from build123d import *

# Parameters (mm, degrees)
CROQUIS2_R              = 1.5
CROQUIS2_R_2            = 1
CROQUIS2_W              = 3
CROQUIS2_H              = 2
SALIENTE_EXTRUIR1_DEPTH = 1


with BuildPart() as part:
    # Croquis2 → Saliente-Extruir1 (new body)
    with BuildSketch(Plane(origin=(0, 0, 0), x_dir=(1, 0, 0), z_dir=(0, 1, 0))):
        Polygon((38, 17), (-3, 17), (-3, 11), (3, 11), (3, 3), (-3, 3), (-3, -3), (15, -3), (15, -6), (20, -6), (20, -3), (38, -3), (38, 3), (32, 3), (32, 11), (38, 11), align=None)
        with Locations(Location((0, 14, 0), (0, 0, 270))):
            Circle(CROQUIS2_R, mode=Mode.SUBTRACT)
        with Locations(Location((0, 0, 0), (0, 0, 270))):
            Circle(CROQUIS2_R, mode=Mode.SUBTRACT)
        with Locations(Location((35, 0, 0), (0, 0, 270))):
            Circle(CROQUIS2_R, mode=Mode.SUBTRACT)
        with Locations(Location((35, 14, 0), (0, 0, 270))):
            Circle(CROQUIS2_R, mode=Mode.SUBTRACT)
        with Locations(Location((17.5, 7, 0), (0, 0, 270))):
            Circle(CROQUIS2_R_2, mode=Mode.SUBTRACT)
        with Locations((17.5, -4)):
            Rectangle(CROQUIS2_W, CROQUIS2_H, mode=Mode.SUBTRACT)
    extrude(amount=SALIENTE_EXTRUIR1_DEPTH)


solid = part.part
Read the model definition and answer for the solid it produces. Units are mm, in the model's axes. A direction names the side the tool comes from. Round coordinates to 2 decimals unless told otherwise and drop trailing zeros. Write each loop counter-clockwise with the first axis right and the second up, starting at its lowest first coordinate (ties: lowest second). Pieces come first, ordered by that corner, then holes. Notation, with made-up numbers: (35.5, 85.25) - (77.5, 85.25) arc R23 cw to (77.5, 94.25) - close; hole circle Ø11 at (87, -12). An arc over 180 degrees is marked (long way). One line per question, with ' | ' between items. Start each with the question number.
1. Each of these flat-tipped pins is pushed along its axis until it touches: pin 1 (1.8 mm diameter, centred on x = 17.5, z = -7, fed in from -Y); pin 2 (0.5 mm diameter, centred on y = 0.5, z = 4, fed in from +X); pin 3 (0.5 mm diameter, centred on x = 0, y = 0.5, fed in from +Z). Where does it stop, or does it pass through?
2. Section C-C (z = 0) is taken. Determine the outline of the cut face in (x, y).
3. Find the intervals of material crossed by probe 1 along X at (y, z) = (0.85, 0); probe 2 along X at (y, z) = (0.75, -7); probe 3 along Z at (x, y) = (1, 0.5), in increasing order. Write a range as [from, to].
4. Section A-A (x = 0) is taken. Determine the outline of the cut face in (y, z).
5. Section B-B (y = 0.2) is taken. Determine the outline of the cut face in (x, z), and give its area (3 significant figures).
6. For faces 1 (the face through (20, 0.5, 4.5)), 2 (the face through (0, 0.5, -11)), 3 (the face through (17.5, 0.5, 5)), 4 (the face through (35, 0.5, -3)), 5 (the face through (5.9, 0.5, 3)), determine the directions among +Z, -Z, +X, -X, +Y, -Y from which every point of the face is accessible in a straight line to the end or side of a thin tool.
7. Section D-D (z = -7) is taken. Determine the outline of the cut face in (x, y), and give its area (3 significant figures).
8. For a pull along X with two mould halves and no side action, classify faces 6 (the face through (28.9, 0.5, 3)), 7 (the face through (-3, 0.5, 0)), 8 (the face through (16, 0.5, 4)) as +X half, -X half, draft (parallel to the pull), parting line (faces both ways), or undercut.
Filled in:
1) pin 1: through | pin 2: x = 20 | pin 3: z = 3
2) outline: (-3, 0) - (-1.5, 0) - (-1.5, 1) - (-3, 1) - close; (1.5, 0) - (33.5, 0) - (33.5, 1) - (1.5, 1) - close; (36.5, 0) - (38, 0) - (38, 1) - (36.5, 1) - close
3) probe 1: [-3, -1.5], [1.5, 33.5], [36.5, 38] | probe 2: [3, 16.5], [18.5, 32] | probe 3: [-17, -15.12], [-12.88, -11], [-3, -1.12], [1.12, 3]
4) outline: (0, -17) - (1, -17) - (1, -15.5) - (0, -15.5) - close; (0, -12.5) - (1, -12.5) - (1, -11) - (0, -11) - close; (0, -3) - (1, -3) - (1, -1.5) - (0, -1.5) - close; (0, 1.5) - (1, 1.5) - (1, 3) - (0, 3) - close
5) outline: (-3, -17) - (38, -17) - (38, -11) - (32, -11) - (32, -3) - (38, -3) - (38, 3) - (20, 3) - (20, 6) - (15, 6) - (15, 3) - (-3, 3) - (-3, -3) - (3, -3) - (3, -11) - (-3, -11) - close; hole circle Ø3 at (0, -14); hole circle Ø3 at (0, 0); hole (16, 3) - (19, 3) - (19, 5) - (16, 5) - close; hole circle Ø2 at (17.5, -7); hole circle Ø3 at (35, -14); hole circle Ø3 at (35, 0) | area: 702 mm²
6) face 1: +Z, +X, +Y, -Y | face 2: -X, +Y, -Y | face 3: +Y, -Y | face 4: +X, +Y, -Y | face 5: +Z, -X, +Y, -Y
7) outline: (3, 0) - (16.5, 0) - (16.5, 1) - (3, 1) - close; (18.5, 0) - (32, 0) - (32, 1) - (18.5, 1) - close | area: 27.0 mm²
8) face 6: draft | face 7: -X half | face 8: undercut
